Verification items for the finished model (mm, model axes). Face numbers are marked on the shaded views. A direction names the side the tool comes from. Round coordinates to 2 decimals unless told otherwise and drop trailing zeros. Order: outer loops, then holes, each group sorted by start corner. A loop starts at its lowest first (then second) coordinate and runs counter-clockwise, first axis right, second up. Notation, with made-up numbers: M 29,-26.75 L 56,-26.75 A18 cw 56,-19.75 Z; hole C 58.5,26 d5. An arc over 180 degrees is marked long. Use one line per item in the form item = value. Start each with the question number.
Item 1: Cross-section at D-D on z = 47.5. Enter the section's corners in (x, y), then the cut area to 3 significant figures.
Item 2: Cross-section at B-B on y = 7.5. Enter the section's corners in (x, z), then the cut area to 3 significant figures.
Item 3: Cross-section at C-C on x = -48. Enter the section's corners in (y, z), then the cut area to 3 significant figures.
Item 4: Release check for a two-part mould opening along X. For the marked faces 3, 4 and 5 record: +X half, -X half, draft (parallel to the pull), parting line (faces both ways), or undercut.
Item 5: Go/stop test with flat-tipped pins: pin 1 Ø8 at (y, z) = (9.5, 39.5) entering from +X; pin 2 Ø4 at (x, y) = (-18, 16.5) entering from -Z; pin 3 Ø6 at (y, z) = (8, 47.5) entering from -X. Record where each tip stops, or that it passes through.
Item 6: Thickness scan on probe 1 along Y at (x, z) = (-79, 41); probe 2 along X at (y, z) = (3.5, 41); probe 3 along Z at (x, y) = (-15, 18.5). Record the ranges inside material, lowest first. Write a range as [from, to].
Item 7: Cross-section at A-A on z = 35.5. Enter the section's corners in (x, y), then the cut area to 3 significant figures.
Item 8: Tool access check on the marked faces 1 and 2. Record the directions out of +Z, -Z, +X, -X, +Y, -Y that give a thin tool (end or side, any length) a straight path to the whole face; none if there is none.
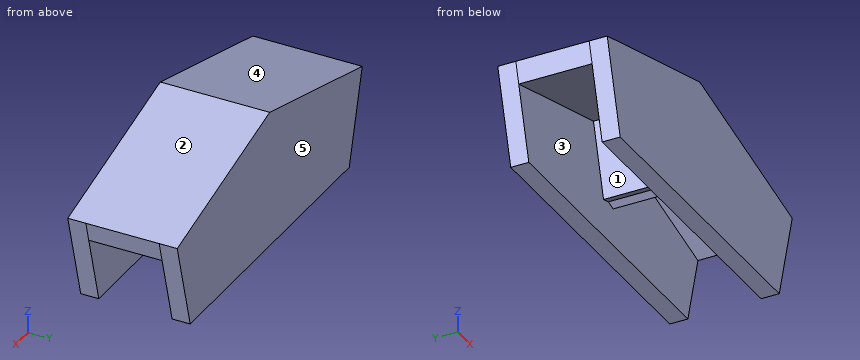
from build123d import *

# Parameters (mm, degrees)
BOSS_EXTRUDE3_DEPTH  = 5
BOSS_EXTRUDE4_DEPTH  = 20.3
BOSS_EXTRUDE5_DEPTH  = 5
BOSS_EXTRUDE16_DEPTH = 5
BOSS_EXTRUDE17_DEPTH = 5


with BuildPart() as part:
    # Sketch4 → Boss-Extrude3 (new body)
    with BuildSketch(Plane(origin=(0, 0, 0), x_dir=(1, 0, 0), z_dir=(0, 1, 0))):
        Polygon((-53.467203663, -64.48008602), (-5.170912349, -51.539133765), (-11.950631556, -26.23687722), (-53.467203663, -37.361209189), (-94.98377577, -26.23687722), (-101.763494978, -51.539133765), align=None)
    extrude(amount=BOSS_EXTRUDE3_DEPTH)

    # Sketch5 → Boss-Extrude4 (add)
    with BuildSketch(Plane(origin=(0, 5, 0), x_dir=(1, 0, 0), z_dir=(0, 1, 0))):
        Polygon((-45.713177048, -56.299630481), (-6.696604941, -45.845171494), (-5.170912349, -51.539133765), (-53.467203663, -64.48008602), (-101.763494978, -51.539133765), (-100.237802385, -45.845171494), (-61.221230279, -56.299630481), (-55.967203663, -36.691336208), (-53.467203663, -37.361209189), (-50.967203663, -36.691336208), align=None)
    extrude(amount=BOSS_EXTRUDE4_DEPTH)

    # Sketch6 → Boss-Extrude5 (add)
    with BuildSketch(Plane(origin=(0, 25.3, 0), x_dir=(1, 0, 0), z_dir=(0, 1, 0))):
        Polygon((-5.170912349, -51.539133765), (-11.950631556, -26.23687722), (-53.467203663, -37.361209189), (-94.98377577, -26.23687722), (-101.763494978, -51.539133765), (-53.467203663, -64.48008602), align=None)
    extrude(amount=BOSS_EXTRUDE5_DEPTH)

    # Sketch20 → Boss-Extrude16 (add)
    with BuildSketch(Plane.XZ.offset(-25.3)):
        Polygon((-94.98377577, 26.23687722), (-11.950631556, 26.23687722), (-53.467203663, 37.361209189), align=None)
    extrude(amount=-BOSS_EXTRUDE16_DEPTH)

    # Sketch21 → Boss-Extrude17 (add)
    with BuildSketch(Plane.XZ):
        Polygon((-11.950631556, 26.23687722), (-53.467203663, 37.361209189), (-94.98377577, 26.23687722), align=None)
    extrude(amount=-BOSS_EXTRUDE17_DEPTH)


solid = part.part
Output values:
q1.outline = M -100.68,0 L -6.25,0 L -6.25,30.3 L -100.68,30.3 Z; hole M -94.06,5 L -58.86,5 L -58.86,25.3 L -94.06,25.3 Z; hole M -48.07,5 L -12.87,5 L -12.87,25.3 L -48.07,25.3 Z
q1.area = 1,430 mm2
q2.outline = M -101.76,51.54 L -100.24,45.85 L -61.22,56.3 L -55.97,36.69 L -53.47,37.36 L -50.97,36.69 L -45.71,56.3 L -6.7,45.85 L -5.17,51.54 L -53.47,64.48 Z
q2.area = 796 mm2
q3.outline = M 0,26.24 L 5,26.24 L 5,47.77 L 25.3,47.77 L 25.3,26.24 L 30.3,26.24 L 30.3,63.02 L 0,63.02 Z
q3.area = 677 mm2
q4.face_3 = undercut
q4.face_4 = -X half
q4.face_5 = draft
q5.pin_1 = -49.14
q5.pin_2 = 48.34
q5.pin_3 = -101.49
q6.probe_1 = [0, 5], [25.3, 30.3]
q6.probe_2 = [-98.94, -7.99]
q6.probe_3 = [48.07, 54.17]
q7.outline = M -97.47,0 L -9.47,0 L -9.47,5 L -97.47,5 Z; M -97.47,25.3 L -9.47,25.3 L -9.47,30.3 L -97.47,30.3 Z
q7.area = 880 mm2
q8.face_1 = -Z
q8.face_2 = +Z, +X, +Y, -Y
